Geometry: see drawing. Coordinates: mm, zero at the bounding-box minimum. A direction names the side the tool comes from. Give positions to 0.01 mm unless a question says otherwise; leave off trailing zeros. Write each loop counter-clockwise with the first axis right and the second up, starting at its lowest first coordinate (ties: lowest second). Pieces come first, ordered by that corner, then holes. Notation, with made-up numbers: (-2, -28.75) -> (28, -28.75) arc R14 cw to (28, -9.75) -> close; hole circle Ø11 at (-15, 68). An arc over 180 degrees is marked (long way). Answer as a JSON object with one key per item and string values. Group by question number.
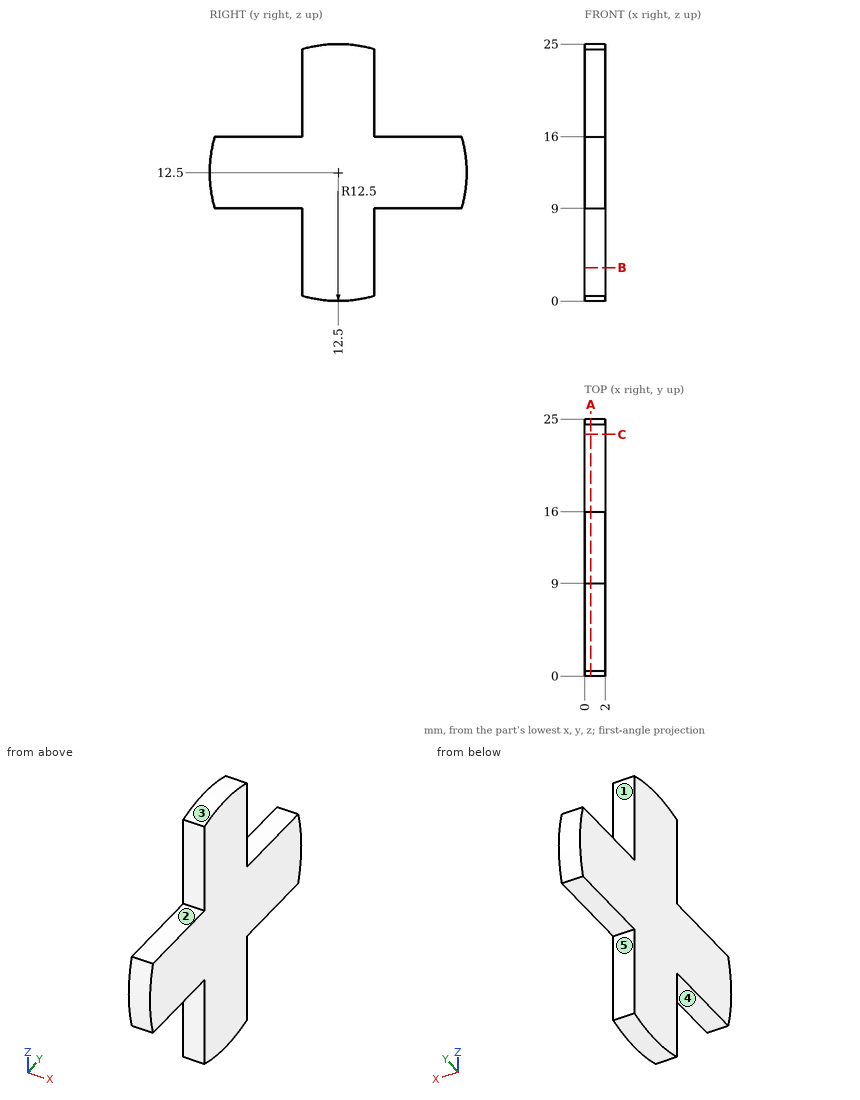
1. Contact query for flat-ended pins moving along their axis: pin 1 Ø1 at (x, z) = (1, 20.5) entering from -Y; pin 2 Ø0.6 at (x, y) = (0.5, 21) entering from +Z; pin 3 Ø1 at (x, z) = (0.5, 11.5) entering from -Y. Output: stop coordinate, or through.
2. Reachability of the marked faces 1, 2, 3, 4 and 5 from +Z, -Z, +X, -X, +Y, -Y: full face, straight path, thin tool, end or side. Return the list, or none.
3. Section B-B (z = 3.25). Return the cut outline in (x, y), plus the area to 3 significant figures.
4. Section A-A (x = 0.6). Return the cut outline in (y, z).
5. Line query: line 1 (Y direction, x = 0.55, z = 3); line 2 (Z direction, x = 1.3, y = 12.5). Output: solid intervals per line, ascending.
Working result:
{
 "1": {"pin 1": "stops at y = 9", "pin 2": "stops at z = 16", "pin 3": "stops at y = 0.01"},
 "2": {"face 1": "+Z, +X, -X, +Y", "face 2": "+Z, +X, -X, -Y", "face 3": "+Z, +X, -X", "face 4": "-Z, +X, -X, -Y", "face 5": "-Z, +X, -X, +Y"},
 "3": {"outline": "(0, 9) -> (2, 9) -> (2, 16) -> (0, 16) -> close", "area": "14.0 mm^2"},
 "4": {"outline": "(0.5, 9) -> (9, 9) -> (9, 0.5) arc R12.5 ccw to (16, 0.5) -> (16, 9) -> (24.5, 9) arc R12.5 ccw to (24.5, 16) -> (16, 16) -> (16, 24.5) arc R12.5 ccw to (9, 24.5) -> (9, 16) -> (0.5, 16) arc R12.5 ccw to start"},
 "5": {"line 1": "y = 9 to 16", "line 2": "z = 0 to 25"}
}
